Autodesk Inventor part; units mm, degrees
ref_plane "YZ Plane" through (0, 0, 0) normal (1, 0, 0) x (0, 1, 0)
ref_plane "XZ Plane" through (0, 0, 0) normal (0, 1, 0) x (-1, 0, 0)
ref_plane "XY Plane" through (0, 0, 0) normal (0, 0, 1) x (1, 0, 0)
sketch "Sketch1" plane through (0, 0, 0) normal (0, 1, 0) x (-1, 0, 0)
  circle A0 centre (0, 0) radius 19.25
  dimension "d0" = 38.5
extrude "Extrusion1" add sketch "Sketch1" along normal blind 93
sketch "Sketch2" plane through (0, 93, 0) normal (0, 1, 0) x (1, 0, 0)
  circle A0 centre (0, 0) radius 19.25
  line L0 (0, 0) -> (33, 0) construction
  line L1 (33, 0) -> (0, 0) construction
  line L2 (0, 0) -> (0, 21) construction
  line L3 (0, 21) -> (33, 21)
  line L4 (33, 21) -> (33, 0)
  line L5 (0, -21) -> (33, -21)
  line L6 (33, -21) -> (33, 0)
  line L7 (0, 21) -> (-33, 21)
  line L8 (-33, 21) -> (-33, 0)
  line L9 (0, -21) -> (-33, -21)
  line L10 (-33, -21) -> (-33, 0)
  dimension "d4" = 33
  dimension "d5" = 21
extrude "Extrusion2" add sketch "Sketch2" along normal blind 42 contours A0 | L3 L4 L6 L5 L9 L10 L8 L7
sketch "Sketch3" plane through (33, 93, 21) normal (1, 0, 0) x (0, 0, -1)
  line L0 (0, 0) -> (42, 0)
  line L1 (42, 0) -> (42, 42)
  line L2 (0, 42) -> (42, 42)
  line L3 (0, 0) -> (0, 42)
  line L4 (0, 42) -> (42, 0) construction
  circle A0 centre (21, 21) radius 16
  point P0 (21, -93)
  dimension "d8" = 32
extrude "Extrusion3" cut sketch "Sketch3" against normal blind 6
move or copy body "Move Body2" bodies to move or copy 1 copy no rotation origin (0, 0, 0) rotation axis (1, 0, 0) rotation angle 90
move or copy body "Move Body4" bodies to move or copy 1 copy no rotation origin (0, 0, 0) rotation axis (0, 0, 1) rotation angle 90
properties part number "Neck_v2"
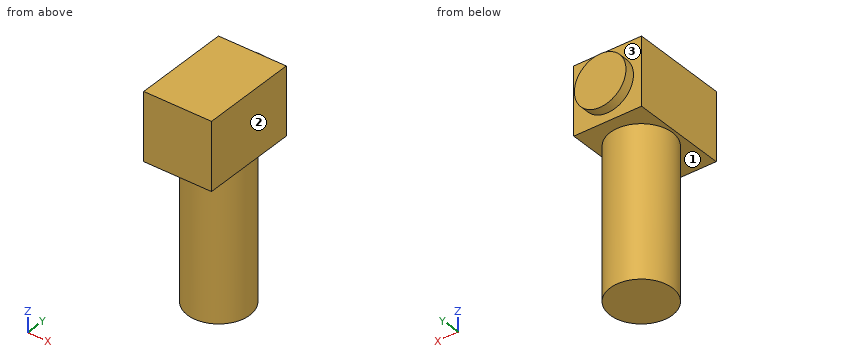
Verification items for the finished model (mm, model axes). Face numbers are marked on the shaded views. A direction names the side the tool comes from. Give positions to 0.01 mm unless a question says otherwise; leave off trailing zeros. Write each loop counter-clockwise with the first axis right and the second up, starting at its lowest first coordinate (ties: lowest second). Pieces come first, ordered by that corner, then holes. Notation, with made-up numbers: M 23,-19.5 L 53,-19.5 A12 cw 53,-5.5 Z; hole C 59,26 d9. An arc over 180 degrees is marked long. Put each result on its own line as item: value. Start each with the question number.
1. Set-up check for the marked faces 1, 2 and 3: record each of +Z, -Z, +X, -X, +Y, -Y from which the full face is reachable in a straight line by a thin tool's end or side.
2. Section check D-D (x = -12). Record the cut outline in (y, z), and give its area (3 significant figures).
3. Section check B-B (y = 0). Record the cut outline in (x, z).
4. Section check A-A (x = 0). Record the cut outline in (y, z).
5. Section check C-C (z = 114). Record the cut outline in (x, y), and give its area (3 significant figures).
6. Scan lines: line 1 along Z through (x, y) = (6.5, -18.5); line 2 along Y through (x, z) = (11, 94.5); line 3 along Y through (x, z) = (15.5, 55). Record each from-to range of solid material in increasing order. Write a range as [from, to].
7. Go/stop test with flat-tipped pins: pin 1 Ø6 at (y, z) = (17.5, 69.5) entering from -X; pin 2 Ø3 at (x, z) = (15.5, 64.5) entering from +Y; pin 3 Ø1 at (y, z) = (-1, 29) entering from -X. Record where each tip stops, or that it passes through.
Answer list:
1. face 1: -Z
1. face 2: +Z, -Z, +X, +Y, -Y
1. face 3: +Y
2. outline: M -33,93 L -15.05,93 L -15.05,0 L 15.05,0 L 15.05,93 L 27,93 L 27,103.42 L 33,103.42 L 33,124.58 L 27,124.58 L 27,135 L -33,135 Z
2. area: 5,450 mm2
3. outline: M -21,93 L -19.25,93 L -19.25,0 L 19.25,0 L 19.25,93 L 21,93 L 21,135 L -21,135 Z
4. outline: M -33,93 L -19.25,93 L -19.25,0 L 19.25,0 L 19.25,93 L 27,93 L 27,98 L 33,98 L 33,130 L 27,130 L 27,135 L -33,135 Z
5. outline: M -21,-33 L 21,-33 L 21,27 L 16,27 L 16,33 L -16,33 L -16,27 L -21,27 Z
5. area: 2,710 mm2
6. line 1: [93, 135]
6. line 2: [-33, 27]
6. line 3: [-11.42, 11.42]
7. pin 1: x = -12.66
7. pin 2: y = 13.21
7. pin 3: x = -19.24
